Input: part model. Units: mm. Frame: model coordinates. A direction names the side the tool comes from. Give positions to 0.01 mm unless a question says otherwise; leave off trailing zeros. Loops run counter-clockwise (first coordinate to the right, second up) from the corner with the lowest first, then second, coordinate; pieces in that order, holes last. Notation, with made-up numbers: (-0.75, -37.75) -> (3.25, -37.75) arc R34 ccw to (3.25, -5.75) -> close; hole circle Ø5 at (40.5, -3). An arc over 180 degrees is marked (long way). Answer as a JSON object with one key per item and string values. Group by question number.
```python
from build123d import *

# Parameters (mm, degrees)
F0_R     = 35
F1_DEPTH = 100
F1_TAPER = -8
F2_T     = -5
F3_R     = 5


with BuildPart() as f1:
    # F0 (on Top) → F1 (new body)
    with BuildSketch(Plane.XY):
        Circle(F0_R)
    extrude(amount=F1_DEPTH, taper=F1_TAPER)

    # F2
    f2_openings = [f1.faces().sort_by_distance(p)[0] for p in [
        (0, 0, 100),
    ]]
    offset(amount=F2_T, openings=f2_openings, kind=Kind.INTERSECTION)

    # F3
    f3_edges = [f1.edges().sort_by_distance(p)[0] for p in [
        (-44.004946, 0, 100),
        (-30.653566, 0, 5),
    ]]
    fillet(f3_edges, radius=F3_R)


solid = f1.part
```
Q1. Set-up query: faces 1 (the face through (0, 0, 0)), 2 (the face through (0, 0, 5)). Return all of +Z, -Z, +X, -X, +Y, -Y with unobstructed straight access to the full face (end or side cutting, diameter ignored); none if empty.
Q2. Pin query (flat end, axial travel): pin 1 Ø10 at (y, z) = (-14, 64) entering from -X; pin 2 Ø3 at (x, z) = (19.5, 26.5) entering from -Y; pin 3 Ø12 at (y, z) = (29.5, 57.5) entering from +X. Return the tip coordinate at first contact, or that it passes through.
Q3. Section A-A on x = 0. Return the cut outline in (y, z), then the cut area to 3 significant figures.
Q4. Ray query, probe 1 along X at (y, z) = (-21, 55.5); probe 2 along X at (y, z) = (31, 84); probe 3 along Y at (x, z) = (22, 88.5). Return the intervals inside material, ascending.
Q5. Section C-C on z = 74. Return the cut outline in (x, y).
Q6. Section B-B on z = 60. Return the cut outline in (x, y).
Numbers:
{
 "1": {"face 1": "-Z, +X, -X, +Y, -Y", "face 2": "+Z"},
 "2": {"pin 1": "stops at x = -43.28", "pin 2": "stops at y = -34.32", "pin 3": "stops at x = 36.23"},
 "3": {"outline": "(-49.05, 100) -> (-35, 0) -> (35, 0) -> (49.05, 100) -> (48.35, 100) arc R5 ccw to (43.4, 95.7) -> (31.26, 9.3) arc R5 cw to (26.31, 5) -> (-26.31, 5) arc R5 cw to (-31.26, 9.3) -> (-43.4, 95.7) arc R5 ccw to (-48.35, 100) -> close", "area": "1,310 mm²"},
 "4": {"probe 1": "x = -37.29 to -31.37, 31.37 to 37.29", "probe 2": "x = -35.07 to -27.97, 27.97 to 35.07", "probe 3": "y = -42.03 to -36.23, 36.23 to 42.03"},
 "5": {"outline": "circle Ø90.8 at (0, 0); hole circle Ø80.7 at (0, 0)"},
 "6": {"outline": "circle Ø86.86 at (0, 0); hole circle Ø76.77 at (0, 0)"}
}
